from build123d import *

# Parameters (mm, degrees)
BOSS_EXTRUDE1_DEPTH = 5


with BuildPart() as part:
    # Sketch1 → Boss-Extrude1 (new body)
    with BuildSketch(Plane.XY):
        with BuildLine():
            Line((-30.63374919, 36.5), (-69, 36.5))
            Line((-69, 36.5), (-69, -30.1))
            Line((-69, -30.1), (-64, -30.1))
            Line((-64, -30.1), (-64, -33.3))
            Line((-64, -33.3), (-61, -33.3))
            Line((-61, -33.3), (-61, -36.5))
            Line((-61, -36.5), (61, -36.5))
            Line((61, -36.5), (61, -33.3))
            Line((61, -33.3), (64, -33.3))
            Line((64, -33.3), (64, -30.1))
            Line((64, -30.1), (69, -30.1))
            Line((69, -30.1), (69, 36.5))
            Line((69, 36.5), (-13.26625081, 36.5))
            ThreePointArc((-13.26625081, 36.5), (-14.828399647, 35.951842978), (-15.7055062, 34.547752809))
            ThreePointArc((-15.7055062, 34.547752809), (-21.95, 29.55), (-28.1944938, 34.547752809))
            ThreePointArc((-28.1944938, 34.547752809), (-29.071600353, 35.951842978), (-30.63374919, 36.5))
        make_face()
        with BuildLine():
            ThreePointArc((3.175, -25.4), (0, -22.225), (-3.175, -25.4))
            ThreePointArc((-3.175, -25.4), (0, -28.575), (3.175, -25.4))
        make_face(mode=Mode.SUBTRACT)
        with BuildLine():
            ThreePointArc((-3.175, 0), (0, -3.175), (3.175, 0))
            ThreePointArc((3.175, 0), (0, 3.175), (-3.175, 0))
        make_face(mode=Mode.SUBTRACT)
        with BuildLine():
            ThreePointArc((-22.225, -25.4), (-25.4, -22.225), (-28.575, -25.4))
            ThreePointArc((-28.575, -25.4), (-25.4, -28.575), (-22.225, -25.4))
        make_face(mode=Mode.SUBTRACT)
        with BuildLine():
            ThreePointArc((28.575, -25.4), (25.4, -22.225), (22.225, -25.4))
            ThreePointArc((22.225, -25.4), (25.4, -28.575), (28.575, -25.4))
        make_face(mode=Mode.SUBTRACT)
        with BuildLine():
            ThreePointArc((-9.525, -12.7), (-12.7, -9.525), (-15.875, -12.7))
            ThreePointArc((-15.875, -12.7), (-12.7, -15.875), (-9.525, -12.7))
        make_face(mode=Mode.SUBTRACT)
        with BuildLine():
            ThreePointArc((-23.3, -12.7), (-25.4, -10.6), (-27.5, -12.7))
            ThreePointArc((-27.5, -12.7), (-25.4, -14.8), (-23.3, -12.7))
        make_face(mode=Mode.SUBTRACT)
        with BuildLine():
            ThreePointArc((14.8, -25.4), (12.7, -23.3), (10.6, -25.4))
            ThreePointArc((10.6, -25.4), (12.7, -27.5), (14.8, -25.4))
        make_face(mode=Mode.SUBTRACT)
        with BuildLine():
            ThreePointArc((-10.6, -25.4), (-12.7, -23.3), (-14.8, -25.4))
            ThreePointArc((-14.8, -25.4), (-12.7, -27.5), (-10.6, -25.4))
        make_face(mode=Mode.SUBTRACT)
        with BuildLine():
            ThreePointArc((2.1, -12.7), (0, -10.6), (-2.1, -12.7))
            ThreePointArc((-2.1, -12.7), (0, -14.8), (2.1, -12.7))
        make_face(mode=Mode.SUBTRACT)
        with BuildLine():
            ThreePointArc((-10.6, 25.4), (-12.7, 27.5), (-14.8, 25.4))
            ThreePointArc((-14.8, 25.4), (-12.7, 23.3), (-10.6, 25.4))
        make_face(mode=Mode.SUBTRACT)
        with BuildLine():
            ThreePointArc((-22.225, 25.4), (-25.4, 28.575), (-28.575, 25.4))
            ThreePointArc((-28.575, 25.4), (-25.4, 22.225), (-22.225, 25.4))
        make_face(mode=Mode.SUBTRACT)
        with BuildLine():
            ThreePointArc((28.575, 25.4), (25.4, 28.575), (22.225, 25.4))
            ThreePointArc((22.225, 25.4), (25.4, 22.225), (28.575, 25.4))
        make_face(mode=Mode.SUBTRACT)
        with BuildLine():
            ThreePointArc((27.5, 12.7), (25.4, 14.8), (23.3, 12.7))
            ThreePointArc((23.3, 12.7), (25.4, 10.6), (27.5, 12.7))
        make_face(mode=Mode.SUBTRACT)
        with BuildLine():
            ThreePointArc((28.575, 0), (25.4, 3.175), (22.225, 0))
            ThreePointArc((22.225, 0), (25.4, -3.175), (28.575, 0))
        make_face(mode=Mode.SUBTRACT)
        with BuildLine():
            ThreePointArc((23.3, -12.7), (25.4, -14.8), (27.5, -12.7))
            ThreePointArc((27.5, -12.7), (25.4, -10.6), (23.3, -12.7))
        make_face(mode=Mode.SUBTRACT)
        with BuildLine():
            ThreePointArc((10.6, 0), (12.7, -2.1), (14.8, 0))
            ThreePointArc((14.8, 0), (12.7, 2.1), (10.6, 0))
        make_face(mode=Mode.SUBTRACT)
        with BuildLine():
            ThreePointArc((9.525, 12.7), (12.7, 9.525), (15.875, 12.7))
            ThreePointArc((15.875, 12.7), (12.7, 15.875), (9.525, 12.7))
        make_face(mode=Mode.SUBTRACT)
        with BuildLine():
            ThreePointArc((10.6, 25.4), (12.7, 23.3), (14.8, 25.4))
            ThreePointArc((14.8, 25.4), (12.7, 27.5), (10.6, 25.4))
        make_face(mode=Mode.SUBTRACT)
        with BuildLine():
            ThreePointArc((3.175, 25.4), (0, 28.575), (-3.175, 25.4))
            ThreePointArc((-3.175, 25.4), (0, 22.225), (3.175, 25.4))
        make_face(mode=Mode.SUBTRACT)
        with BuildLine():
            ThreePointArc((2.1, 12.7), (0, 14.8), (-2.1, 12.7))
            ThreePointArc((-2.1, 12.7), (0, 10.6), (2.1, 12.7))
        make_face(mode=Mode.SUBTRACT)
        with BuildLine():
            ThreePointArc((-27.5, 12.7), (-25.4, 10.6), (-23.3, 12.7))
            ThreePointArc((-23.3, 12.7), (-25.4, 14.8), (-27.5, 12.7))
        make_face(mode=Mode.SUBTRACT)
        with BuildLine():
            ThreePointArc((-9.525, 12.7), (-12.7, 15.875), (-15.875, 12.7))
            ThreePointArc((-15.875, 12.7), (-12.7, 9.525), (-9.525, 12.7))
        make_face(mode=Mode.SUBTRACT)
        with BuildLine():
            ThreePointArc((-10.6, 0), (-12.7, 2.1), (-14.8, 0))
            ThreePointArc((-14.8, 0), (-12.7, -2.1), (-10.6, 0))
        make_face(mode=Mode.SUBTRACT)
        with BuildLine():
            ThreePointArc((9.525, -12.7), (12.7, -15.875), (15.875, -12.7))
            ThreePointArc((15.875, -12.7), (12.7, -9.525), (9.525, -12.7))
        make_face(mode=Mode.SUBTRACT)
        with BuildLine():
            ThreePointArc((-28.575, 0), (-25.4, -3.175), (-22.225, 0))
            ThreePointArc((-22.225, 0), (-25.4, 3.175), (-28.575, 0))
        make_face(mode=Mode.SUBTRACT)
    extrude(amount=-BOSS_EXTRUDE1_DEPTH)


solid = part.part
Geometry: final body of the model. Coordinates: model frame, mm. A direction names the side the tool comes from. Round coordinates to 2 decimals unless told otherwise and drop trailing zeros. Loops run counter-clockwise (first coordinate to the right, second up) from the corner with the lowest first, then second, coordinate; pieces in that order, holes last.
Q1. Pull-direction query (X, two-part tool) for faces 1 (the flat face through (-1, -36.5, -2)), 2 (the cylindrical face through (22.37, -26.35, -2.46)), 3 (the flat face through (-61, -35, -2)); classes: released by +X, released by -X, zero draft, split by the parting line, or undercut.
Q2. Section B-B on y = -25.4. Return loops of the section in (x, z) (3 decimals).
Q3. Section A-A on x = 25.4. Return loops of the section in (y, z) (3 decimals), plus the area to 3 significant figures.
Q4. Access query for faces 4 (the cylindrical face through (-29.053, 35.937, -2.465)), 5 (the cylindrical face through (-22.37, 0.95, -2.46)), 6 (the flat face through (64, -32, -2)). Directions: +Z, -Z, +X, -X, +Y, -Y. A direction counts if a zero-diameter tool reaches every point of the face in a straight line with its end or side. Return the directions, or none.
Q5. Material intervals for L1, parallel to Y at x = -12.7, z = -1.45 (3 decimals); L2, parallel to Y at x = 0, z = -3.2 (3 decimals); L3, parallel to X at y = -14.5, z = -1.5, sorted ascending.
Q6. Section C-C on z = -2.1. State how many separate pieces and enclosed holes the cut face has, plus the area to 3 significant figures.
Q7. Pin query (flat end, axial travel): P1, Ø6, axis at x = 23, y = -2, coming from the +Z side; P2, Ø5, axis at x = -12.7, y = -12.7, coming from the -Z side; P3, Ø1.6, axis at y = -35.5, z = -2, coming from the -X side. Return the tip coordinate at first contact, or that it passes through.
Evaluation:
1. face 1: zero draft
1. face 2: undercut
1. face 3: released by -X
2. outline: (-69, -5) - (-28.575, -5) - (-28.575, 0) - (-69, 0) - close; (-22.225, -5) - (-14.8, -5) - (-14.8, 0) - (-22.225, 0) - close; (-10.6, -5) - (-3.175, -5) - (-3.175, 0) - (-10.6, 0) - close; (3.175, -5) - (10.6, -5) - (10.6, 0) - (3.175, 0) - close; (14.8, -5) - (22.225, -5) - (22.225, 0) - (14.8, 0) - close; (28.575, -5) - (69, -5) - (69, 0) - (28.575, 0) - close
3. outline: (-36.5, -5) - (-28.575, -5) - (-28.575, 0) - (-36.5, 0) - close; (-22.225, -5) - (-14.8, -5) - (-14.8, 0) - (-22.225, 0) - close; (-10.6, -5) - (-3.175, -5) - (-3.175, 0) - (-10.6, 0) - close; (3.175, -5) - (10.6, -5) - (10.6, 0) - (3.175, 0) - close; (14.8, -5) - (22.225, -5) - (22.225, 0) - (14.8, 0) - close; (28.575, -5) - (36.5, -5) - (36.5, 0) - (28.575, 0) - close
3. area: 228 mm2
4. face 4: +Z, -Z, +Y
4. face 5: +Z, -Z
4. face 6: +Z, -Z, +X, -Y
5. L1: y = -36.5 to -27.5, -23.3 to -15.875, -9.525 to -2.1, 2.1 to 9.525, 15.875 to 23.3, 27.5 to 36.5
5. L2: y = -36.5 to -28.575, -22.225 to -14.8, -10.6 to -3.175, 3.175 to 10.6, 14.8 to 22.225, 28.575 to 36.5
5. L3: x = -69 to -26.48, -24.32 to -15.32, -10.08 to -1.08, 1.08 to 10.08, 15.32 to 24.32, 26.48 to 69
6. separate pieces: 1
6. enclosed holes: 25
6. area: 9,340 mm2
7. P1: stops at z = 0
7. P2: passes through
7. P3: stops at x = -61
